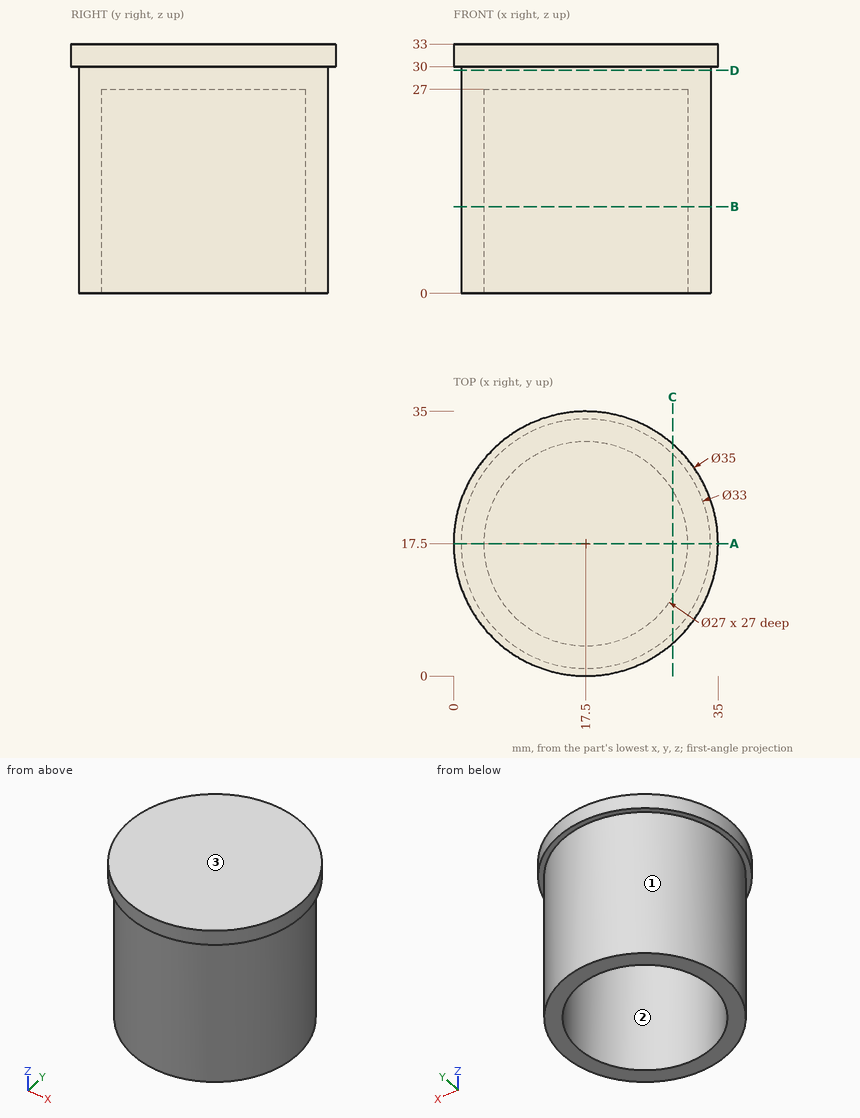
Can you work these out from the drawing? Everything is in mm from the part's minimum corner. Coordinates: 2 decimals unless noted, no trailing zeros. Loops run counter-clockwise (first coordinate to the right, second up) from the corner with the lowest first, then second, coordinate; pieces in that order, holes last.
1. If we mould it in two halves opening along Y, with no side actions, what happens to the marked faces 1, 2 and 3? For each: pulls with the +Y half, pulls with the -Y half, needs draft (parallel to the pull), parting line crosses it, or undercut.
2. I need wall thicknesses on L1, parallel to Y at x = 17.5, z = 19; L2, parallel to Z at x = 23, y = 21.5; L3, parallel to Y at x = 28.5, z = 2.5. Which ranges of each line are inside material? Lowest first, please.
3. Imagine slicing it at D-D, the plane z = 29.5. Please give me the cut outline in (x, y).
4. Imagine slicing it at A-A, the plane y = 17.5. Please give me the cut outline in (x, z), and give its area (3 significant figures).
5. Imagine slicing it at B-B, the plane z = 11.5. Please give me the cut outline in (x, y).
6. For P1, Ø8, axis at y = 31, z = 11, coming from the -X side; P2, Ø4, axis at y = 17, z = 3.5, coming from the -X side; P3, Ø8, axis at x = 8, z = 8.5, coming from the +Y side, each with a flat end and sliding along its axis, tell me the tip position at first contact or that it passes through.
7. Imagine slicing it at C-C, the plane x = 29. Please give me the cut outline in (y, z).
Taken from the geometry:
1. face 1: parting line crosses it
1. face 2: undercut
1. face 3: needs draft
2. L1: y = 1 to 4, 31 to 34
2. L2: z = 27 to 33
2. L3: y = 5.2 to 9.67, 25.33 to 29.8
3. outline: circle Ø33 at (17.5, 17.5)
4. outline: (0, 30) - (1, 30) - (1, 0) - (4, 0) - (4, 27) - (31, 27) - (31, 0) - (34, 0) - (34, 30) - (35, 30) - (35, 33) - (0, 33) - close
4. area: 366 mm2
5. outline: circle Ø33 at (17.5, 17.5); hole circle Ø27 at (17.5, 17.5)
6. P1: stops at x = 4.01
6. P2: stops at x = 1
6. P3: stops at y = 33.06
7. outline: (4.31, 30) - (5.67, 30) - (5.67, 0) - (10.43, 0) - (10.43, 27) - (24.57, 27) - (24.57, 0) - (29.33, 0) - (29.33, 30) - (30.69, 30) - (30.69, 33) - (4.31, 33) - close
